Answer from the drawing. Dimensions are ordinates in mm from the lowest x, y and z of the part. Round coordinates to 2 decimals unless told otherwise and drop trailing zeros. Write each loop counter-clockwise with the first axis right and the second up, starting at its lowest first coordinate (ties: lowest second). Pieces come first, ordered by that corner, then holes. Notation, with made-up numbers: M 83.5,-27.75 L 132.5,-27.75 A25 cw 132.5,-3.75 Z; hole C -25,-17 d1. An arc over 180 degrees is marked long. One line per item, written item: value. Start each with the question number.
(1) Given P1, Ø3, axis at x = 50, z = 5.05, coming from the -Y side, flat-ended and moving along its own axis, determine where the tip first touches the part or whether it passes through.
(2) Section B-B (z = 5.05) is taken. Determine the outline of the cut face in (x, y), plus the area to 3 significant figures.
(3) Consider probe 1 along Z at (x, y) = (50, 4.45); probe 2 along Y at (x, z) = (17, 5.75); probe 3 along X at (y, z) = (2.2, 7.25). Determine where each line is inside the solid, lowest interval first.
(4) Section C-C (y = 1.35) is taken. Determine the outline of the cut face in (x, z).
(5) Section D-D (z = 1.5) is taken. Determine the outline of the cut face in (x, y).
(6) Section A-A (x = 10) is taken. Determine the outline of the cut face in (y, z), plus the area to 3 significant figures.
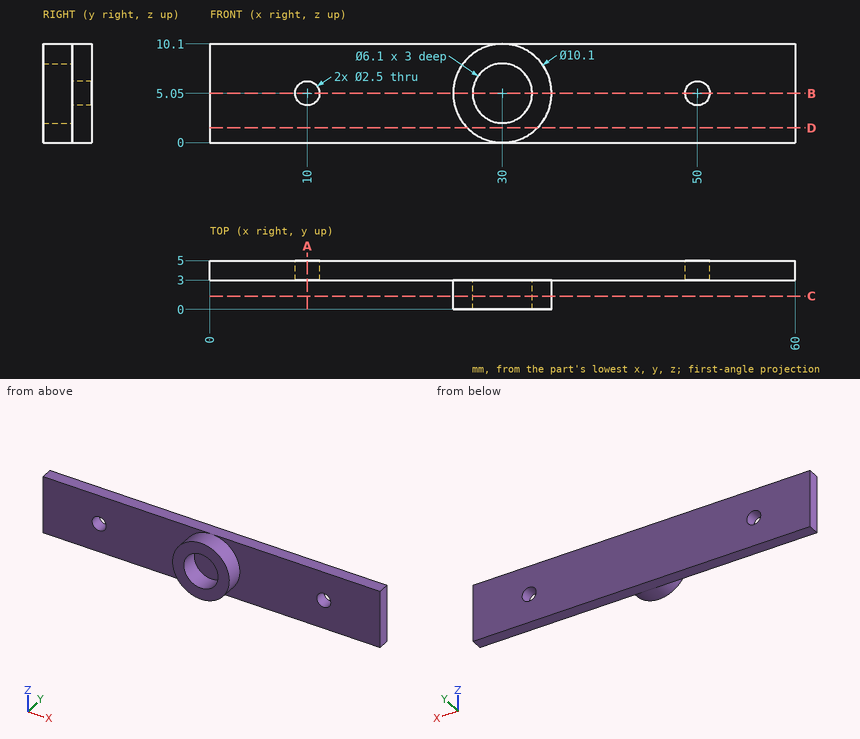
Recorded:
1. P1: stops at y = 3
2. outline: M 0,3 L 8.75,3 L 8.75,5 L 0,5 Z; M 11.25,3 L 24.95,3 L 24.95,0 L 26.95,0 L 26.95,3 L 33.05,3 L 33.05,0 L 35.05,0 L 35.05,3 L 48.75,3 L 48.75,5 L 11.25,5 Z; M 51.25,3 L 60,3 L 60,5 L 51.25,5 Z
2. area: 122 mm2
3. probe 1: z = 0 to 3.8, 6.3 to 10.1
3. probe 2: y = 3 to 5
3. probe 3: x = 25.45 to 27.89, 32.11 to 34.55
4. outline: C 30,5.05 d10.1; hole C 30,5.05 d6.1
5. outline: M 0,3 L 26.41,3 L 26.41,0 L 33.59,0 L 33.59,3 L 60,3 L 60,5 L 0,5 Z
6. outline: M 3,0 L 5,0 L 5,3.8 L 3,3.8 Z; M 3,6.3 L 5,6.3 L 5,10.1 L 3,10.1 Z
6. area: 15.2 mm2
